Verification items for the finished model (mm, model axes). A direction names the side the tool comes from. Give positions to 0.01 mm unless a question says otherwise; leave off trailing zeros. Loops run counter-clockwise (first coordinate to the right, second up) from the corner with the lowest first, then second, coordinate; pieces in that order, holes last. Notation, with made-up numbers: M -7,74.25 L 31,74.25 A35 cw 31,107.25 Z; hole C 29.25,26.5 d5. An arc over 180 degrees is marked long. Use CSV: the item, a comma, the result in double quotes.
from build123d import *

# Parameters (mm, degrees)
F0_W     = 101.6
F0_H     = 76.2
F1_DEPTH = 50.8
F2_SIZE  = 25.4
F4_DEPTH = 76.2
F5_SIZE  = 1.5875
F6_SIZE  = 1.5875


with BuildPart() as f1:
    # F0 (on Front) → F1 (new body, symmetric)
    with BuildSketch(Plane.XZ):
        Rectangle(F0_W, F0_H)
    extrude(amount=F1_DEPTH, both=True)

    # F2
    f2_edges = [f1.edges().sort_by_distance(p)[0] for p in [
        (-50.8, -50.8, 0),
        (0, -50.8, -38.1),
        (50.8, -50.8, 0),
        (0, -50.8, 38.1),
        (-50.8, 50.8, 0),
        (-50.8, 0, -38.1),
        (-50.8, 0, 38.1),
        (0, 50.8, -38.1),
        (50.8, 0, -38.1),
        (50.8, 50.8, 0),
        (50.8, 0, 38.1),
        (0, 50.8, 38.1),
    ]]
    chamfer(f2_edges, length=F2_SIZE)

    # F3 (on Front) → F4 (cut, symmetric)
    with BuildSketch(Plane.XZ):
        Polygon((0, 27.6450640303), (-2.2450640303, 25.4), (0, 23.1549359697), (2.2450640303, 25.4), align=None)
    extrude(amount=F4_DEPTH, both=True, mode=Mode.SUBTRACT)

    # F5
    f5_edges = [f1.edges().sort_by_distance(p)[0] for p in [
        (1.122532, -39.222532, 24.277468),
        (-1.122532, -39.222532, 24.277468),
        (1.122532, 39.222532, 24.277468),
        (-1.122532, 39.222532, 24.277468),
    ]]
    chamfer(f5_edges, length=F5_SIZE)

    # F6
    f6_edges = [f1.edges().sort_by_distance(p)[0] for p in [
        (1.122532, -36.977468, 26.522532),
        (-1.122532, -36.977468, 26.522532),
        (-1.122532, 36.977468, 26.522532),
        (1.122532, 36.977468, 26.522532),
    ]]
    chamfer(f6_edges, length=F6_SIZE)


solid = f1.part
(1) Section check C-C on z = -20.5. Record the cut outline in (x, y).
Calculated:
outline,"M -43,-25.4 L -25.4,-43 L 25.4,-43 L 43,-25.4 L 43,25.4 L 25.4,43 L -25.4,43 L -43,25.4 Z"
(2) Section check B-B on x = -38.5. Record the cut outline in (y, z).
Calculated:
outline,"M -37.7,-12.7 L -25.4,-25 L 25.4,-25 L 37.7,-12.7 L 37.7,12.7 L 25.4,25 L -25.4,25 L -37.7,12.7 Z"
(3) Scan lines: L1, parallel to Y at x = -11, z = -14; L2, parallel to Z at x = 2.5, y = 39.5; L3, parallel to Y at x = -31.5, z = 7. Record each from-to range of solid material in increasing order. Write a range as from..to.
Calculated:
L1,"y = -49.5..49.5"
L2,"z = -24..23.86"
L3,"y = -44.7..44.7"
(4) Mould release check, pull along X, two halves, no side actions. Record for faces 1 (the flat face through (0, -50.8, 0)), 2 (the flat face through (33.1, -33.4, 22.4)), 3 (the flat face through (-1.8, -35.71, 26.81)): released by +X, released by -X, zero draft, split by the parting line, or undercut.
Calculated:
face 1,"zero draft"
face 2,"released by +X"
face 3,"undercut"
(5) Section check D-D on y = 9.5. Record the cut outline in (x, z).
Calculated:
outline,"M -50.8,-12.7 L -25.4,-38.1 L 25.4,-38.1 L 50.8,-12.7 L 50.8,12.7 L 25.4,38.1 L -25.4,38.1 L -50.8,12.7 Z; hole M -2.25,25.4 L 0,23.15 L 2.25,25.4 L 0,27.65 Z"
(6) Depth check by flat-ended pin: pin 1 Ø12 at (y, z) = (26.5, -25.5) entering from +X; pin 2 Ø3 at (y, z) = (-29, 5) entering from -X; pin 3 Ø4 at (x, y) = (-40, -35) entering from +Z. Enter the tip coordinate at first touch or a pass-through.
Calculated:
pin 1,"stops at x = 43.9"
pin 2,"stops at x = -48.7"
pin 3,"stops at z = 16.73"
(7) Section check A-A on y = -28.5. Record the cut outline in (x, z), plus the area to 3 significant figures.
Calculated:
outline,"M -47.7,-12.7 L -25.4,-35 L 25.4,-35 L 47.7,-12.7 L 47.7,12.7 L 25.4,35 L -25.4,35 L -47.7,12.7 Z; hole M -2.25,25.4 L 0,23.15 L 2.25,25.4 L 0,27.65 Z"
area,"5,670 mm²"
(8) Tool access check on faces 4 (the flat face through (1.6, 38.71, 23.8)), 5 (the flat face through (-33.1, -33.4, -22.4)). Record the directions out of +Z, -Z, +X, -X, +Y, -Y that give a thin tool (end or side, any length) a straight path to the whole face; none if there is none.
Calculated:
face 4,"+Z, +Y"
face 5,"-Z, -X, -Y"
